from build123d import *

# Parameters (mm, degrees)
PAD_DEPTH    = 6.7
SKETCH001_W  = 90
SKETCH001_H  = 17.3
PAD001_DEPTH = 0.5


with BuildPart() as part:
    # Sketch (on Sketch) → Pad (new body)
    with BuildSketch(Plane.XY):
        Polygon((-22.7, 3.5), (-2, 3.5), (-2, -3.5), (-22.7, -3.5), (-22.7, -0.6), (-24.7, -0.6), (-24.7, -5.5), (0, -5.5), (0, 5.5), (-24.7, 5.5), (-24.7, 0.6), (-22.7, 0.6), align=None)
    extrude(amount=PAD_DEPTH)

    # Sketch001 → Pad001 (join)
    with BuildSketch(Plane.XY):
        with Locations((-45, 0)):
            Rectangle(SKETCH001_W, SKETCH001_H)
    extrude(amount=-PAD001_DEPTH)


solid = part.part
The listing builds one solid part. Answer for the finished solid, in the listing's coordinates (mm). A direction names the side the tool comes from. Coordinates: 2 decimals unless noted, no trailing zeros. Loops run counter-clockwise (first coordinate to the right, second up) from the corner with the lowest first, then second, coordinate; pieces in that order, holes last. Notation, with made-up numbers: M 31,79.5 L 65,79.5 A12 cw 65,100.5 Z; hole C -31,10.25 d7. An arc over 180 degrees is marked long. Answer in a Markdown table with one row per item.
1) Find section A-A (x = -21.5). Determine the outline of the cut face in (y, z).
Answers below:
| item | result |
|---|---|
| outline | M -8.65,-0.5 L 8.65,-0.5 L 8.65,0 L 5.5,0 L 5.5,6.7 L 3.5,6.7 L 3.5,0 L -3.5,0 L -3.5,6.7 L -5.5,6.7 L -5.5,0 L -8.65,0 Z |
2) Given pin 1 (5 mm diameter, centred on x = -56.5, y = -1, fed in from +Z); pin 2 (4 mm diameter, centred on y = 2.5, z = 4.5, fed in from -X); pin 3 (1 mm diameter, centred on x = -18, z = 5, fed in from +Y), each flat-ended and moving along its own axis, determine where each tip first touches the part or whether it passes through.
Answers below:
| item | result |
|---|---|
| pin 1 | z = 0 |
| pin 2 | x = -24.7 |
| pin 3 | y = 5.5 |
3) Which of the six approach directions +Z, -Z, +X, -X, +Y, -Y give full straight-line access (tool end or side, diameter ignored) to faces 1 (the flat face through (-13, -5.5, 3)), 2 (the flat face through (-24, 0.6, 3)), 3 (the flat face through (-22.7, -2, 3))?
Answers below:
| item | result |
|---|---|
| face 1 | +Z, +X, -X, -Y |
| face 2 | +Z, -X |
| face 3 | +Z |
4) Find section D-D (x = -82). Determine the outline of the cut face in (y, z).
Answers below:
| item | result |
|---|---|
| outline | M -8.65,-0.5 L 8.65,-0.5 L 8.65,0 L -8.65,0 Z |
5) Find section B-B (z = 3.5). Determine the outline of the cut face in (x, y), then the cut area to 3 significant figures.
Answers below:
| item | result |
|---|---|
| outline | M -24.7,-5.5 L 0,-5.5 L 0,5.5 L -24.7,5.5 L -24.7,0.6 L -22.7,0.6 L -22.7,3.5 L -2,3.5 L -2,-3.5 L -22.7,-3.5 L -22.7,-0.6 L -24.7,-0.6 Z |
| area | 124 mm^2 |
6) Find the intervals of material crossed by probe 1 along Y at (x, z) = (-12.5, 1); probe 2 along Z at (x, y) = (-46, 8.25); probe 3 along X at (y, z) = (-1.5, 4), in increasing order.
Answers below:
| item | result |
|---|---|
| probe 1 | -5.5 to -3.5, 3.5 to 5.5 |
| probe 2 | -0.5 to 0 |
| probe 3 | -24.7 to -22.7, -2 to 0 |
7) Determine the mould class of faces 4 (the flat face through (-46, 0, -0.5)), 5 (the flat face through (-2, 0, 3)), 6 (the flat face through (-24.7, 3, 3)) for opening direction X: released by +X, released by -X, zero draft, split by the parting line, or undercut.
Answers below:
| item | result |
|---|---|
| face 4 | zero draft |
| face 5 | undercut |
| face 6 | released by -X |
8) Find section C-C (y = 6.75). Determine the outline of the cut face in (x, z).
Answers below:
| item | result |
|---|---|
| outline | M -90,-0.5 L 0,-0.5 L 0,0 L -90,0 Z |
